Read the model definition and answer for the solid it produces. Units are mm, in the model's axes. Face numbers are marked on the shaded views. A direction names the side the tool comes from. Give positions to 0.01 mm unless a question says otherwise; leave off trailing zeros. Write each loop counter-clockwise with the first axis right and the second up, starting at its lowest first coordinate (ties: lowest second). Pieces come first, ordered by that corner, then holes. Notation, with made-up numbers: (-20, -7) -> (20, -7) arc R12 cw to (20, -2) -> close; hole circle Ø3 at (88.5, -19.5). An arc over 180 degrees is marked (long way). Use a Markdown table: item, result.
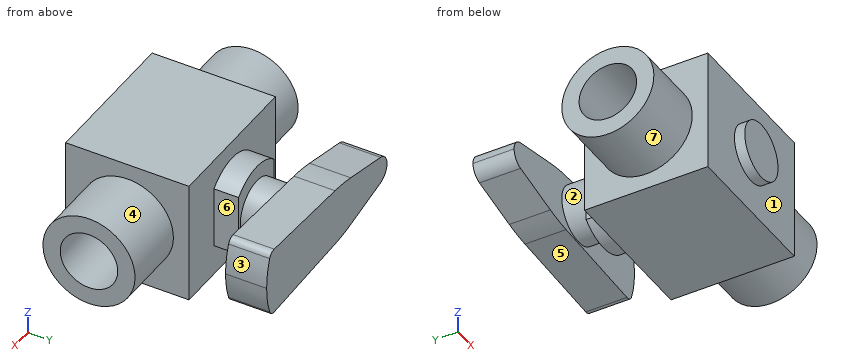
Autodesk Inventor part; units mm, degrees
ref_plane "YZ Plane" through (0, 0, 0) normal (1, 0, 0) x (0, 1, 0)
ref_plane "XZ Plane" through (0, 0, 0) normal (0, 1, 0) x (-1, 0, 0)
ref_plane "XY Plane" through (0, 0, 0) normal (0, 0, 1) x (1, 0, 0)
sketch "Sketch1" plane through (0, 0, 0) normal (0, 0, 1) x (1, 0, 0)
  line L0 (-11.43, 9.525) -> (11.43, 9.525)
  line L1 (11.43, 9.525) -> (11.43, -9.525)
  line L2 (11.43, -9.525) -> (-11.43, -9.525)
  line L3 (-11.43, -9.525) -> (-11.43, 9.525)
  point P0 (0, 0)
  point P1 (-11.43, 0)
  point P2 (0, 9.525)
  dimension "d0" = 19.05
  dimension "d1" = 22.86
extrude "Extrusion1" add sketch "Sketch1" along normal mid plane 19.05
sketch "Sketch2" plane through (-11.43, -9.525, 9.525) normal (-1, 0, 0) x (0, 0, 1)
  line L0 (0, 0) -> (0, 19.05)
  line L1 (-19.05, 19.05) -> (0, 19.05)
  line L2 (-19.05, 19.05) -> (-19.05, 0)
  line L3 (0, 0) -> (-19.05, 0)
  circle A0 centre (-9.525, 9.525) radius 7.112
  point P0 (-9.525, 19.05)
  point P1 (-19.05, 9.525)
  dimension "d4" = 14.224
extrude "Extrusion2" add sketch "Sketch2" along normal blind 10.16 contours A0
sketch "Sketch3" plane through (11.43, -9.525, 9.525) normal (1, 0, 0) x (0, 0, -1)
  circle A0 centre (9.525, 9.525) radius 7.112
  line L0 (0, 19.05) -> (0, 0)
  line L1 (0, 0) -> (19.05, 0)
  line L2 (19.05, 0) -> (19.05, 19.05)
  line L3 (0, 19.05) -> (19.05, 19.05)
  point P0 (9.525, 19.05)
  point P1 (-19.05, 9.525)
  point P2 (0, 9.525)
  point P3 (9.525, 19.05)
  dimension "d7" = 14.224
extrude "Extrusion3" add sketch "Sketch3" along normal blind 10.16 contours A0
sketch "Sketch4" plane through (-11.43, 9.525, 9.525) normal (0, 1, 0) x (1, 0, 0)
  line L0 (0, 0) -> (22.86, 0)
  line L1 (22.86, 0) -> (22.86, 19.05)
  line L2 (22.86, 19.05) -> (0, 19.05)
  line L3 (0, 19.05) -> (0, 0)
  line L4 (16.2654, 14.294) -> (16.2654, 4.756)
  line L5 (6.928, 4.44) -> (6.928, 14.61)
  arc A0 (6.928, 4.44) -> (16.2654, 4.756) centre (11.43, 9.525) ccw
  arc A1 (16.2654, 14.294) -> (6.928, 14.61) centre (11.43, 9.525) ccw
  point P0 (11.43, 19.05)
  point P1 (0, 9.525)
extrude "Extrusion4" add sketch "Sketch4" along normal blind 3.81 contours L4 A0 L5 A1
sketch "Sketch5" plane through (-11.43, 13.335, 9.525) normal (0, 1, 0) x (1, 0, 0)
  arc A0 (6.928, 4.44) -> (16.2654, 4.756) centre (11.43, 9.525) ccw
  line L0 (16.2654, 14.294) -> (16.2654, 4.756)
  arc A1 (16.2654, 14.294) -> (6.928, 14.61) centre (11.43, 9.525) ccw
  line L1 (6.928, 4.44) -> (6.928, 14.61)
  circle A2 centre (11.43, 9.525) radius 4.3993
extrude "Extrusion5" add sketch "Sketch5" along normal blind 10.16 contours A2
sketch "Sketch6" plane through (0, 23.495, 0) normal (0, 1, 0) x (1, 0, 0)
  circle A0 centre (0, 0) radius 4.3993
  line L0 (0, 0) -> (16.7523, 0)
  line L1 (0, 0) -> (-17.0377, 0)
  arc A1 (-15.3253, 2.1404) -> (-17.0377, 0) centre (-14.8437, 0) ccw
  line L2 (-15.3253, 2.1404) -> (-7.4316, 3.9165)
  arc A2 (-3.282, 4.4806) -> (-7.4316, 3.9165) centre (-2.0931, -19.81) ccw
  line L3 (-3.282, 4.4806) -> (12.8089, 5.2681)
  arc A3 (14.0126, 4.4806) -> (12.8089, 5.2681) centre (12.8687, 4.0459) ccw
  arc A4 (14.8116, 0) -> (14.0126, 4.4806) centre (2.5491, 0.1246) ccw
  arc A5 (-17.0377, 0) -> (-15.3253, -2.1404) centre (-14.8437, 0) ccw
  line L4 (-15.3253, -2.1404) -> (-7.4316, -3.9165)
  arc A6 (-7.4316, -3.9165) -> (-3.282, -4.4806) centre (-2.0931, 19.81) ccw
  line L5 (-3.282, -4.4806) -> (12.8089, -5.2681)
  arc A7 (12.8089, -5.2681) -> (14.0126, -4.4806) centre (12.8687, -4.0459) ccw
  arc A8 (14.0126, -4.4806) -> (14.8116, 0) centre (2.5491, -0.1246) ccw
extrude "Extrusion6" add sketch "Sketch6" against normal blind 6.35
sketch "Sketch7" plane through (21.59, 0, 0) normal (1, 0, 0) x (0, 0, -1)
  circle A0 centre (0, 0) radius 4.445
  dimension "d16" = 8.89
extrude "Extrusion7" cut sketch "Sketch7" against normal blind 9.525
sketch "Sketch8" plane through (-21.59, 0, 0) normal (-1, 0, 0) x (0, 0, 1)
  circle A0 centre (0, 0) radius 4.445
  dimension "d19" = 8.89
extrude "Extrusion8" cut sketch "Sketch8" against normal blind 9.525
sketch "Sketch9" plane through (-12.065, 0, 0) normal (-1, 0, 0) x (0, 0, 1)
  circle A0 centre (0, 0) radius 1.5875
  dimension "d23" = 3.175
extrude "Extrusion9" cut sketch "Sketch9" against normal blind 71.4502
thread "Thread1"
thread "Thread2"
sketch "Sketch10" plane through (-11.43, -9.525, 9.525) normal (0, -1, 0) x (1, 0, 0)
  circle A0 centre (11.43, -9.525) radius 4.3993
extrude "Extrusion10" add sketch "Sketch10" along normal blind 1.6002
properties part number "PV609-2"
Item 1: A tool of negligible diameter and unlimited length cuts with its end or side. For the marked faces 4, 5, 6 and 7, from which of +Z, -Z, +X, -X, +Y, -Y can it reach the whole face along a straight path? Write none if from no direction.
Return value:
| item | result |
|---|---|
| face 4 | +X |
| face 5 | -Z, -X, +Y |
| face 6 | +Z, -Z, +X |
| face 7 | -X |
Item 2: For a pull along Y with two mould halves and no side action, classify the marked faces 1, 2 and 3 as +Y half, -Y half, draft (parallel to the pull), parting line (faces both ways), or undercut.
Return value:
| item | result |
|---|---|
| face 1 | -Y half |
| face 2 | undercut |
| face 3 | draft |
Item 3: A cutting plane is placed at C-C (z = 5.75). Give the vertices of the cut face in (x, y) (3 decimals).
Return value:
| item | result |
|---|---|
| outline | (-21.59, -4.185) -> (-11.43, -4.185) -> (-11.43, -9.525) -> (11.43, -9.525) -> (11.43, -4.185) -> (21.59, -4.185) -> (21.59, 4.185) -> (11.43, 4.185) -> (11.43, 9.525) -> (3.614, 9.525) -> (3.614, 13.335) -> (-3.614, 13.335) -> (-3.614, 9.525) -> (-11.43, 9.525) -> (-11.43, 4.185) -> (-21.59, 4.185) -> close |
Item 4: A cutting plane is placed at A-A (y = 0). Give the vertices of the cut face in (x, z) (1 decimal).
Return value:
| item | result |
|---|---|
| outline | (-21.6, -7.1) -> (-11.4, -7.1) -> (-11.4, -9.5) -> (11.4, -9.5) -> (11.4, -7.1) -> (21.6, -7.1) -> (21.6, -4.4) -> (12.1, -4.4) -> (12.1, -1.6) -> (-12.1, -1.6) -> (-12.1, -4.4) -> (-21.6, -4.4) -> close; (-21.6, 4.4) -> (-12.1, 4.4) -> (-12.1, 1.6) -> (12.1, 1.6) -> (12.1, 4.4) -> (21.6, 4.4) -> (21.6, 7.1) -> (11.4, 7.1) -> (11.4, 9.5) -> (-11.4, 9.5) -> (-11.4, 7.1) -> (-21.6, 7.1) -> close |
Item 5: A cutting plane is placed at B-B (x = -9). Give the vertices of the cut face in (y, z) (1 decimal), then the cut area to 3 significant figures.
Return value:
| item | result |
|---|---|
| outline | (-9.5, -9.5) -> (9.5, -9.5) -> (9.5, 9.5) -> (-9.5, 9.5) -> close; (17.1, -3.6) -> (23.5, -3.6) -> (23.5, 3.6) -> (17.1, 3.6) -> close; hole circle Ø3.2 at (0, 0) |
| area | 400 mm^2 |
Item 6: Straight lines are drawn through the part: line 1 along Y through (x, z) = (-9.5, 0) (1 decimal); line 2 along Y through (x, z) = (-15.5, 0) (3 decimals); line 3 along Y through (x, z) = (17, 0) (3 decimals). For each, find the intervals that lie inside material, in ascending order. Write a range as [from, to].
Return value:
| item | result |
|---|---|
| line 1 | [-9.5, -1.6], [1.6, 9.5], [17.1, 23.5] |
| line 2 | [-7.112, -4.445], [4.445, 7.112], [17.145, 23.495] |
| line 3 | [-7.112, -4.445], [4.445, 7.112] |
Item 7: Each of these flat-tipped pins is pushed along its axis until it touches: P1, Ø10, axis at x = -16.5, z = 3, coming from the -Y side; P2, Ø4, axis at x = -12.5, y = -0.5, coming from the -Z side (3 decimals); P3, Ø7, axis at y = 0, z = 0, coming from the -X side (3 decimals); P4, Ø2, axis at y = 16, z = -1.5, coming from the +X side. Where does it stop, or does it pass through?
Return value:
| item | result |
|---|---|
| P1 | y = -7.11 |
| P2 | z = -9.525 |
| P3 | x = -12.065 |
| P4 | x = 4.37 |
